Input: part model. Units: mm. Frame: model coordinates. A direction names the side the tool comes from. Coordinates: 2 decimals unless noted, no trailing zeros. Loops run counter-clockwise (first coordinate to the right, second up) from the corner with the lowest first, then second, coordinate; pieces in that order, holes last. Notation, with made-up numbers: (16, -0.75) -> (35, -0.75) arc R5 ccw to (35, 8.25) -> close; hole circle Ø5 at (-1.75, 11.25). An arc over 180 degrees is marked (long way). Put each result on its own line as item: value. Start each with the question number.
1) Contact query for flat-ended pins moving along their axis: P1, Ø5, axis at y = 7, z = 69, coming from the +X side; P2, Ø2, axis at x = -11, z = 103.5, coming from the +Y side; P3, Ø3, axis at y = 12.5, z = 84.5, coming from the -X side. Output: stop coordinate, or through.
2) Set-up query: faces 1 (the flat face through (-4.4, 12.2, 0)), 2 (the conical face through (16.77, -9.63, -18.65)). Return all of +Z, -Z, +X, -X, +Y, -Y with unobstructed straight access to the full face (end or side cutting, diameter ignored); none if empty.
3) Material intervals for L1, parallel to Z at x = 3, y = -17.5; L2, parallel to X at y = 0.5, z = 134.5; L3, parallel to Z at x = 6, y = 18, sorted ascending.
4) Cut plane A-A (z = 9). Return the cut outline in (x, y), plus the area to 3 significant figures.
from build123d import *

# Parameters (mm, degrees)
F0_R     = 12.7
F1_DEPTH = 177.8
F2_R     = 12.7
F3_DEPTH = 19.05


with BuildPart() as f1:
    # F0 (on Top) → F1 (new body)
    with BuildSketch(Plane.XY):
        Circle(F0_R)
    extrude(amount=F1_DEPTH)

    # F2 (on face) → F3 (join)
    with BuildSketch(Plane(origin=(0, 0, 0), x_dir=(1, 0, 0), z_dir=(0, 0, -1))):
        Polygon((0, -21.5293582698), (18.6449711888, -10.7646791349), (18.6449711888, 10.7646791349), (0, 21.5293582698), (-18.6449711888, 10.7646791349), (-18.6449711888, -10.7646791349), align=None)
        Circle(F2_R, mode=Mode.SUBTRACT)
        Circle(F2_R)
    extrude(amount=F3_DEPTH)

    # F4 (on Front) → F5 (revolve, cut)
    with BuildSketch(Plane.XZ):
        Polygon((31.3791224592, -11.6979343361), (18.6449711888, -19.05), (31.3791224592, -19.05), align=None)
        Polygon((18.6449711888, 0), (31.3791224592, -7.3520656639), (31.3791224592, 0), align=None)
    revolve(axis=Axis((0, 0, -9.525), (0, 0, -1)), mode=Mode.SUBTRACT)


solid = f1.part
Results found:
1. P1: stops at x = 11.88
1. P2: stops at y = 7.83
1. P3: stops at x = -6.35
2. face 1: +Z
2. face 2: -Z, +X, -Y
3. L1: z = -19.05 to 0
3. L2: x = -12.69 to 12.69
3. L3: z = -18.86 to -0.19
4. outline: circle Ø25.4 at (0, 0)
4. area: 507 mm2
